For this review, take the finished solid that the model builds, in its own axes (mm). A direction names the side the tool comes from. Give positions to 0.01 mm unless a question says otherwise; leave off trailing zeros. Write each loop counter-clockwise with the first axis right and the second up, starting at its lowest first coordinate (ties: lowest second). Pieces come first, ordered by that corner, then holes. Notation, with made-up numbers: M 26.5,77 L 59.5,77 A18 ccw 59.5,82 Z; hole C 3,5 d1. An arc over 180 degrees is marked long. Use one line per item in the form item = value. Start each with the question number.
Q1. Consider section C-C on z = 7.5. Write out the cut boundary in (x, y), and give its area (3 significant figures).
Q2. Tool access review of faces 1 (the flat face through (0.87, -0.49, 23.36)), 2 (the flat face through (2, -2, 22)): name each direction out of +Z, -Z, +X, -X, +Y, -Y from which nothing blocks a thin tool from reaching the whole face with its end or side.
Q3. Consider section B-B on y = 1.25. Write out the cut boundary in (x, z), and give its area (3 significant figures).
Q4. Clearance check with flat-ended pins moving along their axes: pin 1 Ø0.6 at (x, z) = (0, 23) entering from -Y; pin 2 Ø2 at (x, y) = (-3.5, 0) entering from -Z; pin 3 Ø5 at (y, z) = (1.5, 10) entering from +X. State where each tip first meets the part, or that it passes through.
Q5. For probe 1 along Y at (x, z) = (0, 13.5); probe 2 along X at (y, z) = (1, 12); probe 3 along X at (y, z) = (2, 3.75), list the stretches that pass through material, from the lowest coordinate up. Write a range as [from, to].
Q6. Consider section D-D on x = 2. Write out the cut boundary in (y, z).
Q7. Consider section A-A on x = 0. Write out the cut boundary in (y, z), and give its area (3 significant figures).
Q8. Mouldability with a two-part tool opening along Y and no side actions: class faces 3 (the flat face through (0, 0, 0)), 4 (the flat face through (0, -1, 23)), 5 (the cylindrical face through (-0.5, -2.4, 10.8)) as released by +Y, released by -Y, zero draft, split by the parting line, or undercut.
```python
from build123d import *

# Parameters (mm, degrees)
SKETCH1_R            = 2.45
BOSS_SHAFT_DEPTH     = 22
SKETCH2_R            = 4.75
BOSS_HEAD_BASE_DEPTH = 0.1
DOME_M5_FACE_RADIUS  = 4.75
DOME_M5_HEIGHT       = 2.75
CUT_HEX_DEPTH        = 3.85


with BuildPart() as part:
    # Sketch1 → Boss-Shaft (new body)
    with BuildSketch(Plane.XY):
        Circle(SKETCH1_R)
    extrude(amount=BOSS_SHAFT_DEPTH)

    # Sketch2 → Boss-Head Base (add)
    with BuildSketch(Plane.XY.offset(22)):
        Circle(SKETCH2_R)
    extrude(amount=BOSS_HEAD_BASE_DEPTH)

    # Dome-M5: a dome of height H over a round flat face of radius A is a cap of a sphere of radius (A * A + H * H) / (2 * H)
    dome_m5_r = (DOME_M5_FACE_RADIUS * DOME_M5_FACE_RADIUS + DOME_M5_HEIGHT * DOME_M5_HEIGHT) / (2 * DOME_M5_HEIGHT)
    dome_m5_base = Plane((0, 0, 22.1), z_dir=(0, 0, 1))
    with Locations(dome_m5_base.offset(DOME_M5_HEIGHT - dome_m5_r)):
        dome_m5_ball = Sphere(dome_m5_r, mode=Mode.PRIVATE)
    add(split(dome_m5_ball, bisect_by=dome_m5_base, keep=Keep.TOP, mode=Mode.PRIVATE))

    # Sketch3 → Cut-Hex (cut, through all)
    with BuildSketch(Plane(origin=(0, 0, 22), x_dir=(-1, 0, 0), z_dir=(0, 0, -1))):
        Polygon((-0.577350269, 1), (-1.154700538, 0), (-0.577350269, -1), (0.577350269, -1), (1.154700538, 0), (0.577350269, 1), align=None)
    extrude(amount=-CUT_HEX_DEPTH, mode=Mode.SUBTRACT)


solid = part.part
```
Working result:
q1.outline = C 0,0 d4.9
q1.area = 18.9 mm²
q2.face_1 = +Z
q2.face_2 = -Z
q3.outline = M -4.58,22 L -2.11,22 L -2.11,0 L 2.11,0 L 2.11,22 L 4.58,22 L 4.58,22.1 A5.33 ccw -4.58,22.1 Z
q3.area = 111 mm²
q4.pin_1 = -4.35
q4.pin_2 = 22
q4.pin_3 = 2.45
q5.probe_1 = [-2.45, 2.45]
q5.probe_2 = [-2.24, 2.24]
q5.probe_3 = [-1.42, 1.42]
q6.outline = M -4.31,22 L -1.42,22 L -1.42,0 L 1.42,0 L 1.42,22 L 4.31,22 L 4.31,22.1 A5.1 ccw -4.31,22.1 Z
q7.outline = M -4.75,22 L -2.45,22 L -2.45,0 L 2.45,0 L 2.45,22 L 4.75,22 L 4.75,22.1 A5.48 ccw 1,24.76 L 1,22 L -1,22 L -1,24.76 A5.48 ccw -4.75,22.1 Z
q7.area = 122 mm²
q8.face_3 = zero draft
q8.face_4 = undercut
q8.face_5 = split by the parting line
